Geometry: final body of the model. Coordinates: model frame, mm. A direction names the side the tool comes from. Give positions to 0.01 mm unless a question says otherwise; leave off trailing zeros. Loops run counter-clockwise (first coordinate to the right, second up) from the corner with the lowest first, then second, coordinate; pieces in that order, holes last. Notation, with made-up numbers: (29, -23.75) - (36, -23.75) arc R14 cw to (36, -4.75) - close; hole circle Ø3 at (19.5, 41). An arc over 180 degrees is marked (long way). Answer in a Markdown table with one row per item.
from build123d import *
from build123d.topology import SkipClean

# Parameters (mm, degrees)
SKETCH1_R             = 1.9
SKETCH1_R_2           = 4.25
SKETCH1_R_3           = 1.1
BOSS_EXTRUDE1_DEPTH   = 5
SKETCH4_R             = 1.75
CUT_EXTRUDE3_DEPTH    = 2.25
CORTAR_EXTRUIR1_DEPTH = 10
REDONDEO1_R           = 10
CHAFL_N1_SIZE         = 0.75


with BuildPart() as part:
    # Sketch1 → Boss-Extrude1 (new body)
    with BuildSketch(Plane.XY):
        with BuildLine():
            Line((-18.558111277, 4.616096398), (-25.278111277, -18.423903602))
            ThreePointArc((-25.278111277, -18.423903602), (-14.718111277, -32.503903602), (-4.158111277, -18.423903602))
            Line((-4.158111277, -18.423903602), (-10.878111277, 4.616096398))
            ThreePointArc((-10.878111277, 4.616096398), (-14.718111277, 7.496096398), (-18.558111277, 4.616096398))
        make_face()
        with Locations((-14.718111277, 3.496096398)):
            Circle(SKETCH1_R, mode=Mode.SUBTRACT)
        with Locations((-14.718111277, -21.503903602)):
            Circle(SKETCH1_R_2, mode=Mode.SUBTRACT)
        with Locations((-6.718111277, -21.503903602)):
            Circle(SKETCH1_R_3, mode=Mode.SUBTRACT)
        with Locations((-9.061257027, -27.160757851)):
            Circle(SKETCH1_R_3, mode=Mode.SUBTRACT)
        with Locations((-14.718111277, -29.503903602)):
            Circle(SKETCH1_R_3, mode=Mode.SUBTRACT)
        with Locations((-20.374965526, -27.160757851)):
            Circle(SKETCH1_R_3, mode=Mode.SUBTRACT)
        with Locations((-22.718111277, -21.503903602)):
            Circle(SKETCH1_R_3, mode=Mode.SUBTRACT)
        with Locations((-20.374965526, -15.847049352)):
            Circle(SKETCH1_R_3, mode=Mode.SUBTRACT)
        with Locations((-14.718111277, -13.503903602)):
            Circle(SKETCH1_R_3, mode=Mode.SUBTRACT)
        with Locations((-9.061257027, -15.847049352)):
            Circle(SKETCH1_R_3, mode=Mode.SUBTRACT)
    extrude(amount=BOSS_EXTRUDE1_DEPTH)

    # Sketch4 → Cut-Extrude3 (cut)
    with BuildSketch(Plane(origin=(0, 0, 0), x_dir=(-1, 0, 0), z_dir=(0, 0, -1))):
        with Locations((22.718111277, -21.503903602)):
            Circle(SKETCH4_R)
        with Locations((20.374965526, -27.160757851)):
            Circle(SKETCH4_R)
        with Locations((14.718111277, -29.503903602)):
            Circle(SKETCH4_R)
        with Locations((9.061257027, -27.160757851)):
            Circle(SKETCH4_R)
        with Locations((6.718111277, -21.503903602)):
            Circle(SKETCH4_R)
        with Locations((9.061257027, -15.847049352)):
            Circle(SKETCH4_R)
        with Locations((14.718111277, -13.503903602)):
            Circle(SKETCH4_R)
        with Locations((20.374965526, -15.847049352)):
            Circle(SKETCH4_R)
    extrude(amount=-CUT_EXTRUDE3_DEPTH, mode=Mode.SUBTRACT)

    # Croquis1 → Cortar-Extruir1 (cut)
    with SkipClean():  # the faces are left unmerged after this step: merging them gives an invalid solid
        with BuildSketch(Plane(origin=(0, 0, 0), x_dir=(-1, 0, 0), z_dir=(0, 0, -1))):
            with BuildLine():
                Line((10.719078773, 3.408124606), (11.039054977, -11.13739287))
                ThreePointArc((11.039054977, -11.13739287), (6.720549727, -13.951486157), (4.158111277, -18.423903602))
                Line((4.158111277, -18.423903602), (10.878111277, 4.616096398))
                ThreePointArc((10.878111277, 4.616096398), (10.752331831, 4.018201167), (10.719078773, 3.408124606))
            make_face()
        extrude(amount=-CORTAR_EXTRUIR1_DEPTH, mode=Mode.SUBTRACT)

    # Redondeo1
    redondeo1_edges = [part.edges().sort_by_distance(p)[0] for p in [
        (-11.039054977, -11.13739287, 2.5),
    ]]
    fillet(redondeo1_edges, radius=REDONDEO1_R)

    # Chaflán1
    chafl_n1_edges = [part.edges().sort_by_distance(p)[0] for p in [
        (-10.816579688, -1.024083907, 0),
        (-10.06427699, -9.715796647, 0),
        (-14.718111277, -32.503903602, 0),
        (-21.918111277, -6.903903602, 0),
        (-14.718111277, 7.496096398, 0),
    ]]
    chamfer(chafl_n1_edges, length=CHAFL_N1_SIZE)


solid = part.part
Q1. Material intervals for line 1 along Y through (x, z) = (-7.5, 0.7); line 2 along X through (y, z) = (-27.5, 2.2); line 3 along X through (y, z) = (-27, 4.55), sorted ascending.
Check values:
| item | result |
|---|---|
| line 1 | -29.74 to -27.95, -26.37 to -23.07, -19.94 to -16.64, -15.06 to -13.27 |
| line 2 | -23.94 to -22.09, -18.66 to -10.78, -7.34 to -5.5 |
| line 3 | -24.25 to -21.46, -19.29 to -10.15, -7.97 to -5.19 |
Q2. Cut plane B-B (y = -3). Output: boundary loops of the cut face in (x, z).
Check values:
| item | result |
|---|---|
| outline | (-20.78, 0.75) - (-20, 0) - (-11.61, 0) - (-10.86, 0.75) - (-10.86, 5) - (-20.78, 5) - close |
Q3. First-contact query: pin 1 (2 mm diameter, centred on x = -20.37, y = -15.85, fed in from -Z); pin 2 (2 mm diameter, centred on x = -23, z = 3, fed in from -Y); pin 3 (4 mm diameter, centred on x = -14, y = -29, fed in from -Z); pin 4 (1.7 mm diameter, centred on x = -15.5, y = -13.5, fed in from -Z). Flat tips, straight axial feed; report the tip coordinate or a pass-through.
Check values:
| item | result |
|---|---|
| pin 1 | through |
| pin 2 | y = -29.75 |
| pin 3 | z = 0 |
| pin 4 | z = 2.25 |
Q4. Cut plane A-A (z = 4.4). Give the number of separate pieces and of enclosed holes in the cut face, and give its area (3 significant figures).
Check values:
| item | result |
|---|---|
| separate pieces | 1 |
| enclosed holes | 10 |
| area | 466 mm² |
Q5. Reachability of faces 1 (the cylindrical face through (-10.04, -9.77, 2.9)), 2 (the cylindrical face through (-6.957, -22.578, 3.606)), 3 (the cylindrical face through (-13.43, -12.32, 1.11)) from +Z, -Z, +X, -X, +Y, -Y: full face, straight path, thin tool, end or side. Return the list, or none.
Check values:
| item | result |
|---|---|
| face 1 | +Z, -Z, +X |
| face 2 | +Z, -Z |
| face 3 | -Z |
Q6. Draft query along Y for faces 4 (the flat face through (-21.61, -7.17, 0.38)), 5 (the cylindrical face through (-14.861, -28.413, 3.606)), 6 (the flat face through (-8, -17, 2.25)), 7 (the flat face through (-15, -17, 5)). Return one class per face: pulls with the +Y half, pulls with the -Y half, needs draft (parallel to the pull), parting line crosses it, or undercut.
Check values:
| item | result |
|---|---|
| face 4 | pulls with the +Y half |
| face 5 | undercut |
| face 6 | undercut |
| face 7 | needs draft |
